Read the model definition and answer for the solid it produces. Units are mm, in the model's axes. Give positions to 0.01 mm unless a question says otherwise; leave off trailing zeros. Write each loop counter-clockwise with the first axis right and the second up, starting at its lowest first coordinate (ties: lowest second). Pieces come first, ordered by that corner, then holes. Notation, with made-up numbers: (83.5, 22.25) -> (92.5, 22.25) arc R20 ccw to (92.5, 61.25) -> close; hole circle Ø5 at (5.25, 45.5). An arc over 180 degrees is marked (long way). Use a Markdown table: item, result.
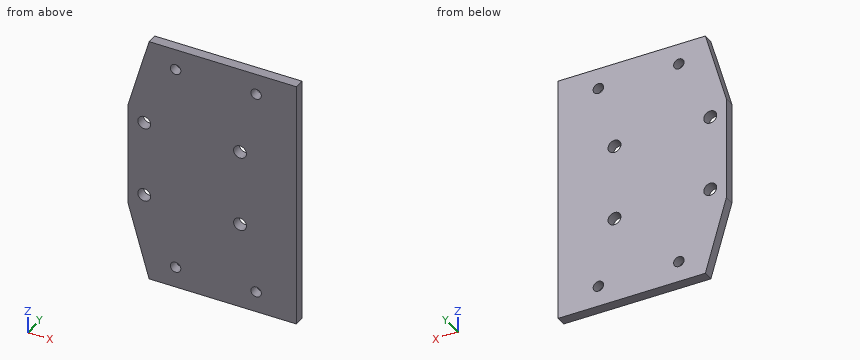
from build123d import *

# Parameters (mm, degrees)
SKETCH1_W           = 57.15
SKETCH1_H           = 79.248
BOSS_EXTRUDE1_DEPTH = 3.175
SKETCH2_R           = 1.651
CUT_EXTRUDE1_DEPTH  = 79.095767635
SKETCH3_R           = 2.032
CUT_EXTRUDE2_DEPTH  = 79.095767635
CUT_EXTRUDE3_DEPTH  = 79.095767635


with BuildPart() as part:
    # Sketch1 → Boss-Extrude1 (new body)
    with BuildSketch(Plane(origin=(0, 0, 0), x_dir=(1, 0, 0), z_dir=(0, 1, 0))):
        with Locations((-26.398757506, -15.754283497)):
            Rectangle(SKETCH1_W, SKETCH1_H)
    extrude(amount=-BOSS_EXTRUDE1_DEPTH)

    # Sketch2 → Cut-Extrude1 (cut, through all)
    with BuildSketch(Plane(origin=(0, 0, 0), x_dir=(1, 0, 0), z_dir=(0, 1, 0))):
        with Locations(Location((-35.923757506, -48.774283497, 0), (0, 0, 270))):
            Circle(SKETCH2_R)
        with Locations(Location((-35.923757506, 17.265716503, 0), (0, 0, 270))):
            Circle(SKETCH2_R)
        with Locations(Location((-10.523757506, -48.774283497, 0), (0, 0, 270))):
            Circle(SKETCH2_R)
        with Locations(Location((-10.523757506, 17.265716503, 0), (0, 0, 270))):
            Circle(SKETCH2_R)
    extrude(amount=-CUT_EXTRUDE1_DEPTH, mode=Mode.SUBTRACT)

    # Sketch3 → Cut-Extrude2 (cut, through all)
    with BuildSketch(Plane(origin=(0, 0, 0), x_dir=(1, 0, 0), z_dir=(0, 1, 0))):
        with Locations(Location((-45.829757506, -3.689283497, 0), (0, 0, 270))):
            Circle(SKETCH3_R)
        with Locations(Location((-15.603757506, -3.689283497, 0), (0, 0, 270))):
            Circle(SKETCH3_R)
        with Locations(Location((-45.829757506, -27.819283497, 0), (0, 0, 270))):
            Circle(SKETCH3_R)
        with Locations(Location((-15.603757506, -27.819283497, 0), (0, 0, 270))):
            Circle(SKETCH3_R)
    extrude(amount=-CUT_EXTRUDE2_DEPTH, mode=Mode.SUBTRACT)

    # Sketch4 → Cut-Extrude3 (cut, through all)
    with BuildSketch(Plane(origin=(0, 0, 0), x_dir=(1, 0, 0), z_dir=(0, 1, 0))):
        Polygon((-50.909757506, -32.264283497), (-50.909757506, 0.755716503), (-40.921106308, 35.590282968), (-90.515991817, 35.590282968), (-90.515991817, -67.098849962), (-50.909757506, -67.098849962), (-40.921106308, -67.098849962), align=None)
    extrude(amount=-CUT_EXTRUDE3_DEPTH, mode=Mode.SUBTRACT)


solid = part.part
Item 1: Straight lines are drawn through the part: line 1 along Z through (x, y) = (-14, -2.5); line 2 along X through (y, z) = (-1.65, 26); line 3 along X through (y, z) = (-0.2, 2.5). For each, find the intervals that lie inside material, in ascending order. Write a range as [from, to].
Return value:
| item | result |
|---|---|
| line 1 | [-23.87, 2.44], [4.94, 26.57], [29.07, 55.38] |
| line 2 | [-50.91, -46.73], [-44.92, -16.51], [-14.7, 2.18] |
| line 3 | [-50.91, -47.48], [-44.18, -17.25], [-13.96, 2.18] |
Item 2: Each of these flat-tipped pins is pushed along its axis until it touches: P1, Ø3, axis at x = -10.52, z = -17.27, coming from the -Y side; P2, Ø4, axis at x = -35.92, z = 48.77, coming from the +Y side. Where does it stop, or does it pass through?
Return value:
| item | result |
|---|---|
| P1 | through |
| P2 | y = 0 |
Item 3: A cutting plane is placed at C-C (z = -7.5). Give the vertices of the cut face in (x, y) (3 decimals), then the cut area to 3 significant figures.
Return value:
| item | result |
|---|---|
| outline | (-48.976, -3.175) -> (2.176, -3.175) -> (2.176, 0) -> (-48.976, 0) -> close |
| area | 162 mm^2 |
Item 4: A cutting plane is placed at A-A (y = -1.4). Count the separate pieces of the cut face and the enclosed holes in it, then the cut area to 3 significant figures.
Return value:
| item | result |
|---|---|
| separate pieces | 1 |
| enclosed holes | 8 |
| area | 3,970 mm^2 |
Item 5: A cutting plane is placed at B-B (z = 37). Give the vertices of the cut face in (x, y) (3 decimals).
Return value:
| item | result |
|---|---|
| outline | (-49.552, -3.175) -> (2.176, -3.175) -> (2.176, 0) -> (-49.552, 0) -> close |
